from build123d import *

# Parameters (mm, degrees)
SKETCH_1_W      = 29
SKETCH_1_H      = 20
EXTRUDE_1_DEPTH = 24
SKETCH_2_W      = 14.5
SKETCH_2_H      = 10
SKETCH_2_W_2    = 5.5
EXTRUDE_2_DEPTH = 10
EXTRUDE_3_DEPTH = 30


with BuildPart() as part:
    # 草图1 → 凸台-拉伸1 (new body)
    with BuildSketch(Plane(origin=(0, 0, 0), x_dir=(1, 0, 0), z_dir=(0, 1, 0))):
        with Locations((14.5, 10)):
            Rectangle(SKETCH_1_W, SKETCH_1_H)
    extrude(amount=EXTRUDE_1_DEPTH)

    # 草图2 → 凸台-拉伸2 (add)
    with BuildSketch(Plane(origin=(0, 24, 0), x_dir=(1, 0, 0), z_dir=(0, 1, 0))):
        with Locations((7.25, 5)):
            Rectangle(SKETCH_2_W, SKETCH_2_H)
        Polygon((0, 0), (0, 10), (0, 20), (14.5, 20), (29, 20), (29, 10), (34.5, 10), (34.5, 25), (-5.5, 25), (-5.5, -5), (34.5, -5), (34.5, 0), (29, 0), (14.5, 0), align=None)
        with Locations((21.75, 5)):
            Rectangle(SKETCH_2_W, SKETCH_2_H)
        with Locations((31.75, 5)):
            Rectangle(SKETCH_2_W_2, SKETCH_2_H)
        with Locations((21.75, 15)):
            Rectangle(SKETCH_2_W, SKETCH_2_H)
        with Locations((7.25, 15)):
            Rectangle(SKETCH_2_W, SKETCH_2_H)
    extrude(amount=EXTRUDE_2_DEPTH)

    # 草图3 → 凸台-拉伸3 (add)
    with BuildSketch(Plane(origin=(0, 34, 0), x_dir=(1, 0, 0), z_dir=(0, 1, 0))):
        with BuildLine():
            ThreePointArc((14.5, 20), (7.428932188, 17.071067812), (4.5, 10))
            Line((4.5, 10), (14.5, 10))
            Line((14.5, 10), (14.5, 20))
        make_face()
        with BuildLine():
            Line((14.5, 10), (4.5, 10))
            ThreePointArc((4.5, 10), (7.428932188, 2.928932188), (14.5, 0))
            Line((14.5, 0), (14.5, 10))
        make_face()
        with BuildLine():
            Line((14.5, 20), (14.5, 10))
            Line((14.5, 10), (24.5, 10))
            ThreePointArc((24.5, 10), (21.571067812, 17.071067812), (14.5, 20))
        make_face()
        with BuildLine():
            Line((24.5, 10), (14.5, 10))
            Line((14.5, 10), (14.5, 0))
            ThreePointArc((14.5, 0), (21.571067812, 2.928932188), (24.5, 10))
        make_face()
    extrude(amount=EXTRUDE_3_DEPTH)


solid = part.part
Could you check a few things on this model? Use its own coordinates, in mm. A direction names the side the tool comes from. Give positions to 0.01 mm unless a question says otherwise; leave off trailing zeros. Write each loop counter-clockwise with the first axis right and the second up, starting at its lowest first coordinate (ties: lowest second). Pieces come first, ordered by that corner, then holes. Notation, with made-up numbers: (24.5, 87.25) -> (71.5, 87.25) arc R26 cw to (71.5, 105.25) -> close; hole circle Ø6 at (-10, 14.5). An arc over 180 degrees is marked (long way). Write each question's results on one line, items separated by ' | '. Start each with the question number.
Q1. Suppose I cut it at A-A, the plane x = 9. List the corners of the cut face in (y, z) for me, and give its area (3 significant figures).
Q2. Which directions (+Z, -Z, +X, -X, +Y, -Y) give clear straight access to the entire face, cutting with the end or side of a thin tool? Please do faces 1 (the face through (29, 12, -10)), 2 (the face through (0, 12, -10)), 3 (the face through (14, 12, -20)), 4 (the face through (14.2, 34, -20.2)).
Q3. I'm going to push flat-ended pins straight in: pin 1 Ø16 at (y, z) = (8.5, -11) entering from +X; pin 2 Ø2 at (x, y) = (27, 13.5) entering from +Z; pin 3 Ø6 at (x, y) = (29, 49) entering from -Z; pin 4 Ø4 at (x, y) = (13, 35.5) entering from +Z. Where does each tip first touch, or does it pass through?
Q4. Suppose I cut it at D-D, the plane y = 15.5. List the corners of the cut face in (x, z) for me.
Q5. Suppose I cut it at C-C, the plane y = 45. List the corners of the cut face in (x, z) for me, and give its area (3 significant figures).
Q6. Suppose I cut it at B-B, the plane z = -1.75. List the corners of the cut face in (x, y) for me.
Q7. I need wall thicknesses on probe 1 along X at (y, z) = (23, -6.75); probe 2 along Y at (x, z) = (32.5, -22.5); probe 3 along Z at (x, y) = (15.5, 9.5). Which ranges of each line are inside material? Lowest first, please.
Outcome:
1) outline: (0, -20) -> (24, -20) -> (24, -25) -> (34, -25) -> (34, -18.35) -> (64, -18.35) -> (64, -1.65) -> (34, -1.65) -> (34, 5) -> (24, 5) -> (24, 0) -> (0, 0) -> close | area: 1,280 mm2
2) face 1: +Z, -Z, +X, -Y | face 2: +Z, -Z, -X, -Y | face 3: -Z, +X, -X, -Y | face 4: +Y
3) pin 1: x = 29 | pin 2: z = 0 | pin 3: through | pin 4: z = 5
4) outline: (0, -20) -> (29, -20) -> (29, 0) -> (0, 0) -> close
5) outline: circle Ø20 at (14.5, -10) | area: 314 mm2
6) outline: (-5.5, 24) -> (0, 24) -> (0, 0) -> (29, 0) -> (29, 24) -> (34.5, 24) -> (34.5, 34) -> (20.15, 34) -> (20.15, 64) -> (8.85, 64) -> (8.85, 34) -> (-5.5, 34) -> close
7) probe 1: 0 to 29 | probe 2: 24 to 34 | probe 3: -20 to 0
